Verification items for the finished model (mm, model axes). A direction names the side the tool comes from. Coordinates: 2 decimals unless noted, no trailing zeros. Loops run counter-clockwise (first coordinate to the right, second up) from the corner with the lowest first, then second, coordinate; pieces in that order, holes last. Notation, with made-up numbers: M 39,-39.5 L 60,-39.5 A23 cw 60,-21.5 Z; hole C 85.5,15 d5. An arc over 180 degrees is marked long. Write item = value, one per line. Start each with the question number.
Autodesk Inventor part; units mm, degrees
ref_plane "YZ Plane" through (0, 0, 0) normal (1, 0, 0) x (0, 1, 0)
ref_plane "XZ Plane" through (0, 0, 0) normal (0, 1, 0) x (-1, 0, 0)
ref_plane "XY Plane" through (0, 0, 0) normal (0, 0, 1) x (1, 0, 0)
sketch "Sketch1" plane through (0, 0, 0) normal (0, 1, 0) x (-1, 0, 0)
  line L0 (0, 0) -> (0, -4.7) construction
  line L1 (3.5, 0) -> (-3.5, 0) construction
  line L2 (3.5, 0) -> (3.5, -6.55) construction
  line L3 (3.5, -6.55) -> (2.5, -6.55)
  line L4 (-3.5, -6.55) -> (-2.5, -6.55)
  arc A0 (2.5, -6.55) -> (-2.5, -6.55) centre (0, -7.3142) ccw
  line L5 (3.5, -2.05) -> (-3.5, -2.05)
  line L6 (3.5, -2.05) -> (3.5, -6.55)
  line L7 (-3.5, -2.05) -> (-3.5, -6.55)
  dimension "d0" = 4.7
  dimension "d1" = 7
  dimension "d2" = 3.5
  dimension "d3" = 6.55
  dimension "d4" = 1
  dimension "d5" = 1
  dimension "d6" = 2.05
revolve "Revolution1" add sketch "Sketch1" angle 360 about axis through (-3.5, 0, 0) along (1, 0, 0)
sketch "Sketch2" plane through (-3.5, 0, 0) normal (-1, 0, 0) x (0, 0, 1)
  circle A0 centre (0, 0) radius 6.55
  circle A1 centre (0, 0) radius 2.05
  circle A2 centre (0, 0) radius 2.65
  circle A3 centre (0, 0) radius 3.85
  point P0 (0, 0)
  dimension "d8" = 5.3
  dimension "d9" = 7.7
extrude "Extrusion1" cut sketch "Sketch2" against normal blind 1 contours A3
sketch "Sketch3" plane through (3.5, 0, 0) normal (1, 0, 0) x (0, 0, -1)
  circle A0 centre (0, 0) radius 3.85
  circle A1 centre (0, 0) radius 2.65
  dimension "d12" = 7.7
  dimension "d13" = 5.3
extrude "Extrusion2" cut sketch "Sketch3" against normal blind 1
equation "\"d2\" = 0.5 * d1"
properties part number "WheelYBottom"
Q1. Gauge pin test, flat ends, axial feed: pin 1 (3 mm diameter, centred on x = 2, y = 4, fed in from -Z); pin 2 (4 mm diameter, centred on x = -3, y = -5, fed in from -Z); pin 3 (4 mm diameter, centred on x = -1, y = 3.5, fed in from +Z). Record the tip position at first contact, or that the pin passes through.
Q2. Sectioned sample at A-A on z = 0. Record the cut outline in (x, y), plus the area to 3 significant figures.
Q3. Set-up check for faces 1 (the face through (-3.01, -3.76, -0.83)), 2 (the face through (3.5, -2, -1)), 3 (the face through (3.01, -3.76, 0.83)): record each of +Z, -Z, +X, -X, +Y, -Y from which the full face is reachable in a straight line by a thin tool's end or side.
Q4. Sectioned sample at D-D on x = 1.75. Record the cut outline in (y, z), plus the area to 3 significant figures.
Q5. Mould release check, pull along Z, two halves, no side actions. Record for faces 4 (the face through (3.5, -3, -3)), 5 (the face through (2.5, -3, 1)), 6 (the face through (2.993, -6.494, 0.853)): +Z half, -Z half, draft (parallel to the pull), parting line (faces both ways), or undercut.
Q6. Sectioned sample at C-C on x = -2.75. Record the cut outline in (y, z).
Q7. Scan lines: L1, parallel to Y at x = -3, z = 0; L2, parallel to Z at x = -2.75, y = 0.5; L3, parallel to X at y = -5.5, z = -3.25. Record each from-to range of solid material in increasing order. Write a range as [from, to].
Solutions:
q1.pin_1 = -6.02
q1.pin_2 = -5.82
q1.pin_3 = 6.18
q2.outline = M -3.5,-6.55 L -2.5,-6.55 A2.61 cw 2.5,-6.55 L 3.5,-6.55 L 3.5,-3.85 L 2.5,-3.85 L 2.5,-2.65 L 3.5,-2.65 L 3.5,-2.05 L -3.5,-2.05 L -3.5,-2.65 L -2.5,-2.65 L -2.5,-3.85 L -3.5,-3.85 Z; M -3.5,2.05 L 3.5,2.05 L 3.5,2.65 L 2.5,2.65 L 2.5,3.85 L 3.5,3.85 L 3.5,6.55 L 2.5,6.55 A2.61 cw -2.5,6.55 L -3.5,6.55 L -3.5,3.85 L -2.5,3.85 L -2.5,2.65 L -3.5,2.65 Z
q2.area = 44.6 mm²
q3.face_1 = -X
q3.face_2 = +Z, -Z, +X, +Y, -Y
q3.face_3 = +X
q4.outline = C 0,0 d10.74; hole C 0,0 d4.1
q4.area = 77.5 mm²
q5.face_4 = draft
q5.face_5 = undercut
q5.face_6 = parting line
q6.outline = C 0,0 d13.1; C 0,0 d5.3; hole C 0,0 d7.7; hole C 0,0 d4.1
q7.L1 = [-6.55, -3.85], [-2.65, -2.05], [2.05, 2.65], [3.85, 6.55]
q7.L2 = [-6.53, -3.82], [-2.6, -1.99], [1.99, 2.6], [3.82, 6.53]
q7.L3 = [-3.5, -2.44], [2.44, 3.5]
